Work out the finished part from the listing and answer in its coordinate system (mm). Face numbers are marked on the shaded views. A direction names the side the tool comes from. Round coordinates to 2 decimals unless told otherwise and drop trailing zeros. Order: outer loops, then holes, each group sorted by start corner. A loop starts at its lowest first (then second) coordinate and runs counter-clockwise, first axis right, second up. Notation, with made-up numbers: (26, 89) - (50, 89) arc R29 cw to (50, 116) - close; hole circle Ø8 at (88, 52.5). An arc over 180 degrees is marked (long way). Answer in a Markdown table with one row per item.
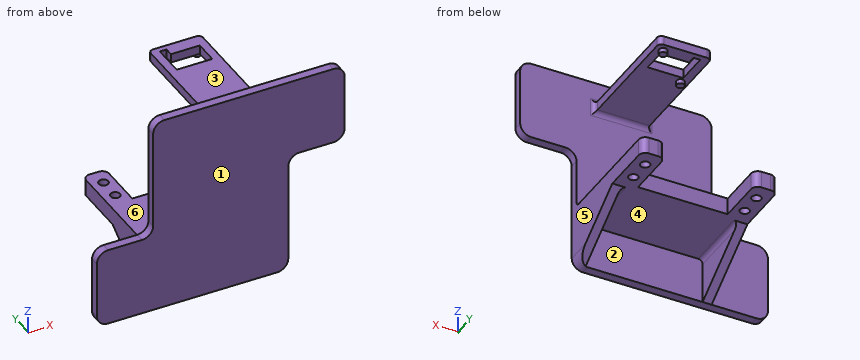
from build123d import *

# Parameters (mm, degrees)
SKETCH2_W                = 60
SKETCH2_H                = 55
BOSS_EXTRUDE1_DEPTH      = 7.5
SKETCH3_W                = 39.8
SKETCH3_H                = 45
CUT_EXTRUDE1_DEPTH       = 42.382363393
SKETCH4_R                = 2.1
CUT_EXTRUDE2_DEPTH       = 42.382363393
BOSS_EXTRUDE2_DEPTH      = 3
BOSS_EXTRUDE2_DEPTH_BACK = 1
SKETCH6_R                = 1.7
SKETCH6_W                = 15.8
SKETCH6_H                = 10.5
SKETCH7_W                = 3
SKETCH7_H                = 3.7
CUT_EXTRUDE3_DEPTH       = 4
SKETCH8_R                = 1.7
BOSS_EXTRUDE4_DEPTH      = 6
SKETCH10_W               = 60
SKETCH10_H               = 89
BOSS_EXTRUDE5_DEPTH      = 4
BOSS_EXTRUDE6_DEPTH      = 4
LPATTERN1_COUNT          = 2
LPATTERN1_PITCH          = 56
FILLET1_R                = 3
FILLET3_R                = 2
FILLET4_R                = 2
FILLET5_R                = 2
FILLET6_R                = 2
FILLET7_R                = 2
FILLET8_R                = 2
FILLET9_R                = 2
FILLET10_R               = 2
SKETCH12_W               = 25
SKETCH12_H               = 35
BOSS_EXTRUDE7_DEPTH      = 4
FILLET11_R               = 5


with BuildPart() as part:
    # Sketch2 → Boss-Extrude1 (new body)
    with BuildSketch(Plane.XY):
        Rectangle(SKETCH2_W, SKETCH2_H)
    extrude(amount=BOSS_EXTRUDE1_DEPTH)

    # Sketch3 → Cut-Extrude1 (cut, through all)
    with BuildSketch(Plane.XY.offset(7.5)):
        with Locations((0, 27.5)):
            Rectangle(SKETCH3_W, SKETCH3_H)
    extrude(amount=-CUT_EXTRUDE1_DEPTH, mode=Mode.SUBTRACT)

    # Sketch4 → Cut-Extrude2 (cut, through all)
    with BuildSketch(Plane.XY.offset(7.5)):
        with Locations((-24.71, 20.03)):
            Circle(SKETCH4_R)
        with Locations((-24.71, 10.18)):
            Circle(SKETCH4_R)
        with Locations(Location((24.71, 20.03, 0), (0, 0, 180))):
            Circle(SKETCH4_R)
        with Locations(Location((24.71, 10.18, 0), (0, 0, 180))):
            Circle(SKETCH4_R)
    extrude(amount=-CUT_EXTRUDE2_DEPTH, mode=Mode.SUBTRACT)



with BuildPart() as body_2:
    # Sketch6 → Boss-Extrude2 (new, two sides: drawn at the far end of the back side and taken through both)
    with BuildSketch(Plane.XY.offset(56).offset(-BOSS_EXTRUDE2_DEPTH_BACK)):
        Polygon((-1.45, 3.4), (-1.45, 26.3), (21.75, 26.3), (21.75, 3.4), (21.75, -27.5), (-1.45, -27.5), align=None)
        with Locations((18.194, 22.744)):
            Circle(SKETCH6_R, mode=Mode.SUBTRACT)
        with Locations((2.11, 6.956)):
            Circle(SKETCH6_R, mode=Mode.SUBTRACT)
        with Locations((10.15, 14.85)):
            Rectangle(SKETCH6_W, SKETCH6_H, mode=Mode.SUBTRACT)
    extrude(amount=BOSS_EXTRUDE2_DEPTH + BOSS_EXTRUDE2_DEPTH_BACK)

    # Sketch7 → Cut-Extrude3 (cut)
    with BuildSketch(Plane.XY.offset(59)):
        with Locations((3.75, 21.95)):
            Rectangle(SKETCH7_W, SKETCH7_H)
    extrude(amount=-CUT_EXTRUDE3_DEPTH, mode=Mode.SUBTRACT)

    # Sketch8 → Boss-Extrude4 (add)
    with BuildSketch(Plane.XY.offset(59)):
        with Locations((18.194, 22.744)):
            Circle(SKETCH8_R)
        with Locations((2.11, 6.956)):
            Circle(SKETCH8_R)
    extrude(amount=-BOSS_EXTRUDE4_DEPTH)


with BuildPart() as part_1:
    add(part.part)

    add(body_2.part)  # Boss-Extrude5 merges body 2
    # Sketch10 → Boss-Extrude5 (add)
    with BuildSketch(Plane.XZ.offset(27.5)):
        with Locations((0, 24.5)):
            Rectangle(SKETCH10_W, SKETCH10_H)
    extrude(amount=BOSS_EXTRUDE5_DEPTH)

    # Sketch11 → Boss-Extrude6 (add)
    with BuildSketch(Plane(origin=(30, 0, 0), x_dir=(0, 0, -1), z_dir=(1, 0, 0))):
        Polygon((0, 2.5), (20, -27.5), (0, -27.5), align=None)
    boss_extrude6 = extrude(amount=-BOSS_EXTRUDE6_DEPTH)

    # LPattern1: Boss-Extrude6 ×2
    with Locations(*[(-i * LPATTERN1_PITCH, 0, 0) for i in range(1, LPATTERN1_COUNT)]):
        add(boss_extrude6)

    # Fillet1
    fillet1_edges = [part_1.edges().sort_by_distance(p)[0] for p in [
        (19.9, 27.5, 3.75),
        (-19.9, 27.5, 3.75),
        (-30, 27.5, 3.75),
        (30, 27.5, 3.75),
    ]]
    fillet(fillet1_edges, radius=FILLET1_R)

    # Fillet3
    fillet3_edges = [part_1.edges().sort_by_distance(p)[0] for p in [
        (21.75, 26.3, 57),
        (-1.45, 26.3, 57),
    ]]
    fillet(fillet3_edges, radius=FILLET3_R)

    # Fillet4
    fillet4_edges = [part_1.edges().sort_by_distance(p)[0] for p in [
        (-1.45, -27.5, 57),
    ]]
    fillet(fillet4_edges, radius=FILLET4_R)

    # Fillet5
    fillet5_edges = [part_1.edges().sort_by_distance(p)[0] for p in [
        (21.75, -27.5, 57),
    ]]
    fillet(fillet5_edges, radius=FILLET5_R)

    # Fillet6
    fillet6_edges = [part_1.edges().sort_by_distance(p)[0] for p in [
        (0, -27.5, 7.5),
    ]]
    fillet(fillet6_edges, radius=FILLET6_R)

    # Fillet7
    fillet7_edges = [part_1.edges().sort_by_distance(p)[0] for p in [
        (10.15, -27.5, 55),
    ]]
    fillet(fillet7_edges, radius=FILLET7_R)

    # Fillet8
    fillet8_edges = [part_1.edges().sort_by_distance(p)[0] for p in [
        (10.15, -27.5, 59),
    ]]
    fillet(fillet8_edges, radius=FILLET8_R)

    # Fillet9
    fillet9_edges = [part_1.edges().sort_by_distance(p)[0] for p in [
        (26, -12.5, 0),
    ]]
    fillet(fillet9_edges, radius=FILLET9_R)

    # Fillet10
    fillet10_edges = [part_1.edges().sort_by_distance(p)[0] for p in [
        (-26, -12.5, 0),
    ]]
    fillet(fillet10_edges, radius=FILLET10_R)

    # Sketch12 → Boss-Extrude7 (add)
    with BuildSketch(Plane.XZ.offset(31.5)):
        with Locations((-42.5, -2.5)):
            Rectangle(SKETCH12_W, SKETCH12_H)
        with Locations((42.5, 51.5)):
            Rectangle(SKETCH12_W, SKETCH12_H)
    extrude(amount=-BOSS_EXTRUDE7_DEPTH)

    # Fillet11
    # the kernel refuses this fillet: 5 mm, written as the material it adds along each edge
    with BuildSketch(Plane(origin=(-30, -31.5, 15), x_dir=(-1, 0, 0), z_dir=(0, 1, 0)), Plane(origin=(30, -31.5, 34), x_dir=(1, 0, 0), z_dir=(0, 1, 0))) as fillet11_piece_1:
        with BuildLine():
            CenterArc((FILLET11_R, FILLET11_R), FILLET11_R, 180, 90)
            Line((0, FILLET11_R), (0, 0))
            Line((0, 0), (FILLET11_R, 0))
        make_face()
    extrude(amount=4)
    # the kernel refuses this fillet: 5 mm, written as the material it takes off along each edge
    with BuildSketch(Plane(origin=(-55, -44, 15), x_dir=(0, 0, -1), z_dir=(0, 1, 0)), Plane(origin=(-55, -44, -20), x_dir=(1, 0, 0), z_dir=(0, 1, 0)), Plane(origin=(30, -15, -20), x_dir=(-1, 0, 0), z_dir=(0, -1, 0))) as fillet11_2_piece_1:
        with BuildLine():
            CenterArc((FILLET11_R, -FILLET11_R), FILLET11_R, 90, 90)
            Line((0, -FILLET11_R), (0, 0))
            Line((0, 0), (FILLET11_R, 0))
        make_face()
    extrude(amount=29, mode=Mode.SUBTRACT)
    with BuildSketch(Plane(origin=(55, -44, 34), x_dir=(-1, 0, 0), z_dir=(0, 1, 0)), Plane(origin=(55, -44, 69), x_dir=(0, 0, -1), z_dir=(0, 1, 0)), Plane(origin=(-30, -15, 69), x_dir=(0, 0, -1), z_dir=(0, -1, 0))) as fillet11_2_piece_2:
        with BuildLine():
            CenterArc((FILLET11_R, FILLET11_R), FILLET11_R, 180, 90)
            Line((0, FILLET11_R), (0, 0))
            Line((0, 0), (FILLET11_R, 0))
        make_face()
    extrude(amount=29, mode=Mode.SUBTRACT)


solid = part_1.part
1) Which of the six approach directions +Z, -Z, +X, -X, +Y, -Y give full straight-line access (tool end or side, diameter ignored) to the marked faces 1, 2 and 3?
Filled in:
| item | result |
|---|---|
| face 1 | +Z, -Z, +X, -X, -Y |
| face 2 | -Z, +Y |
| face 3 | +Z, +X, -X, +Y |
2) Find section B-B, the plane z = 1.5. Give the vertices of the cut face in (x, y).
Filled in:
| item | result |
|---|---|
| outline | (-55, -31.5) - (30, -31.5) - (30, 24.5) arc R3 ccw to (27, 27.5) - (22.9, 27.5) arc R3 ccw to (19.9, 24.5) - (19.9, 5) - (-19.9, 5) - (-19.9, 24.5) arc R3 ccw to (-22.9, 27.5) - (-27, 27.5) arc R3 ccw to (-30, 24.5) - (-30, -27.5) - (-55, -27.5) - close; hole circle Ø4.2 at (-24.71, 10.18); hole circle Ø4.2 at (-24.71, 20.03); hole circle Ø4.2 at (24.71, 10.18); hole circle Ø4.2 at (24.71, 20.03) |
3) Find section C-C, the plane z = -13. Give the vertices of the cut face in (x, y), then the cut area to 3 significant figures.
Filled in:
| item | result |
|---|---|
| outline | (-55, -31.5) - (30, -31.5) - (30, -17) - (26, -17) - (26, -27.5) - (-26, -27.5) - (-26, -17) - (-30, -17) - (-30, -27.5) - (-55, -27.5) - close |
| area | 424 mm^2 |
4) Find section D-D, the plane y = -23.5. Give the vertices of the cut face in (x, z), then the cut area to 3 significant figures.
Filled in:
| item | result |
|---|---|
| outline | (-30, -17.33) - (-26, -17.33) - (-26, -2) arc R2 cw to (-24, 0) - (24, 0) arc R2 cw to (26, -2) - (26, -17.33) - (29.42, -17.33) arc R5 ccw to (30, -15) - (30, 7.5) - (-30, 7.5) - close; (-1.45, 55) - (21.75, 55) - (21.75, 59) - (-1.45, 59) - close |
| area | 683 mm^2 |
5) Find the intervals of material crossed by probe 1 along Y at (x, z) = (24.71, 6); probe 2 along X at (y, z) = (10, 2); probe 3 along X at (y, z) = (-26, -7.5), in increasing order. Write a range as from..to.
Filled in:
| item | result |
|---|---|
| probe 1 | y = -31.5..8.08, 12.28..17.93, 22.13..27.5 |
| probe 2 | x = -30..-26.8, -22.62..-19.9, 19.9..22.62, 26.8..30 |
| probe 3 | x = -30..-26, 26..30 |
6) The mould has two halves that part along X. Classify the marked faces 4, 5 and 6: released by +X, released by -X, zero draft, split by the parting line, or undercut.
Filled in:
| item | result |
|---|---|
| face 4 | undercut |
| face 5 | released by +X |
| face 6 | zero draft |
7) Find section A-A, the plane y = -15.5. Give the vertices of the cut face in (x, z).
Filled in:
| item | result |
|---|---|
| outline | (-30, -12) - (-26, -12) - (-26, -2) arc R2 cw to (-24, 0) - (24, 0) arc R2 cw to (26, -2) - (26, -12) - (30, -12) - (30, 7.5) - (-30, 7.5) - close; (-1.45, 55) - (21.75, 55) - (21.75, 59) - (-1.45, 59) - close |
8) Each of these flat-tipped pins is pushed along its axis until it touches: pin 1 (3 mm diameter, centred on y = -3.5, z = 58, fed in from -X); pin 2 (5.5 mm diameter, centred on x = 24.71, y = 10.18, fed in from -Z); pin 3 (3 mm diameter, centred on x = -45.5, y = -30, fed in from +Z); pin 4 (4 mm diameter, centred on x = 24.71, y = 20.03, fed in from -Z). Where does it stop, or does it pass through?
Filled in:
| item | result |
|---|---|
| pin 1 | stops at x = -1.45 |
| pin 2 | stops at z = 0 |
| pin 3 | stops at z = 15 |
| pin 4 | passes through |
